Source: CAD feature listing. Evaluate the final solid. Frame: model axes, mm. A direction names the side the tool comes from. Coordinates: 2 decimals unless noted, no trailing zeros. Loops run counter-clockwise (first coordinate to the right, second up) from the corner with the lowest first, then second, coordinate; pieces in that order, holes last.
Item 1: Section query D-D, the plane z = 10.5. Return the cut outline in (x, y).
Item 2: Reachability of faces 1 (the flat face through (-190, -5, -1)), 2 (the cylindrical face through (-239.859, -4.93, 40.746)) from +Z, -Z, +X, -X, +Y, -Y: full face, straight path, thin tool, end or side. Return the list, or none.
Item 3: Pin query (flat end, axial travel): pin 1 Ø2 at (y, z) = (-7.5, 38.5) entering from +X; pin 2 Ø3 at (x, y) = (29.5, -2) entering from +Z; pin 3 Ø3 at (y, z) = (-5.5, 9) entering from -X. Return the tip coordinate at first contact, or that it passes through.
Item 4: Section query C-C, the plane x = 72. Return the cut outline in (y, z), then the cut area to 3 significant figures.
Item 5: Section query B-B, the plane y = -4.5. Return the cut outline in (x, z), then the cut area to 3 significant figures.
Item 6: Pull-direction query (X, two-part tool) for faces 3 (the flat face through (3, -5, 50)), 4 (the flat face through (257, -5, -16)), 5 (the flat face through (-229, -5, -31.778)); classes: +X half, -X half, draft (parallel to the pull), parting line (faces both ways), or undercut.
Item 7: Section query A-A, the plane z = -12.5. Return the cut outline in (x, y), then the cut area to 3 significant figures.
Item 8: Line query: probe 1 along X at (y, z) = (-3.75, -19); probe 2 along Z at (x, y) = (75, -2.5); probe 3 along X at (y, z) = (-8.5, 22). Output: solid intervals per line, ascending.
```python
from build123d import *

# Parameters (mm, degrees)
F1_DEPTH = 10


with BuildPart() as f1:
    # F0 (on Front) → F1 (new body)
    with BuildSketch(Plane.XZ):
        with BuildLine():
            Line((-200, 50), (-200, 57))
            ThreePointArc((-200, 57), (-240.305087, 40.305087), (-257, 0))
            Line((-257, 0), (-257, -31.777661))
            Line((-257, -31.777661), (-200, -31.777661))
            Line((-200, -31.777661), (-200, 0))
            Line((-200, 0), (-200, 28.5))
            Line((-200, 28.5), (-190, 28.5))
            Line((-190, 28.5), (-190, 0))
            Line((-190, 0), (-190, -31.777661))
            Line((-190, -31.777661), (190, -31.777661))
            Line((190, -31.777661), (200, -31.777661))
            Line((200, -31.777661), (257, -31.777661))
            Line((257, -31.777661), (257, 0))
            ThreePointArc((257, 0), (240.305087, 40.305087), (200, 57))
            Line((200, 57), (200, 50))
            Line((200, 50), (-200, 50))
        make_face()
    extrude(amount=F1_DEPTH)


solid = f1.part
```
Verdict:
1. outline: (-256.02, -10) - (-200, -10) - (-200, 0) - (-256.02, 0) - close; (-190, -10) - (256.02, -10) - (256.02, 0) - (-190, 0) - close
2. face 1: -Z, +Y, -Y
2. face 2: +Z, -X, +Y, -Y
3. pin 1: stops at x = 242.93
3. pin 2: stops at z = 50
3. pin 3: stops at x = -256.5
4. outline: (-10, -31.78) - (0, -31.78) - (0, 50) - (-10, 50) - close
4. area: 818 mm2
5. outline: (-257, -31.78) - (-200, -31.78) - (-200, 28.5) - (-190, 28.5) - (-190, -31.78) - (257, -31.78) - (257, 0) arc R57 ccw to (200, 57) - (200, 50) - (-200, 50) - (-200, 57) arc R57 ccw to (-257, 0) - close
5. area: 40,800 mm2
6. face 3: undercut
6. face 4: +X half
6. face 5: draft
7. outline: (-257, -10) - (-200, -10) - (-200, 0) - (-257, 0) - close; (-190, -10) - (257, -10) - (257, 0) - (-190, 0) - close
7. area: 5,040 mm2
8. probe 1: x = -257 to -200, -190 to 257
8. probe 2: z = -31.78 to 50
8. probe 3: x = -252.58 to -200, -190 to 252.58
